Verification items for the finished model (mm, model axes). A direction names the side the tool comes from. Coordinates: 2 decimals unless noted, no trailing zeros. Order: outer loops, then holes, each group sorted by start corner. A loop starts at its lowest first (then second) coordinate and runs counter-clockwise, first axis right, second up.
Q1. Cross-section at C-C, the plane x = 1.1. Count the separate pieces of the cut face and the enclosed holes in it, and give its area (3 significant figures).
Q2. Draft check along Z on faces 1 (the flat face through (2, -65, -40)), 2 (the flat face through (2, -39, 65)), 3 (the cylindrical face through (2, -64, -63)), 4 (the cylindrical face through (1.972, -41.777, 22.704)). Enter one of: pulls with the +Z half, pulls with the -Z half, needs draft (parallel to the pull), parting line crosses it, or undercut.
Q3. Depth check by flat-ended pin: P1, Ø11.5, axis at y = 0, z = -55, coming from the -X side; P2, Ø2, axis at x = 2.5, y = 35, coming from the +Z side; P3, Ø2, axis at x = 1.5, z = -19, coming from the -Y side; P4, Ø1.5, axis at x = 0.5, z = 17, coming from the +Y side. Enter the tip coordinate at first touch or a pass-through.
Q4. Thickness scan on line 1 (Y direction, x = 0.3, z = 36); line 2 (Y direction, x = 0.6, z = 37); line 3 (Y direction, x = 2.45, z = -55). Record the ranges inside material, lowest first.
Q5. Set-up check for faces 5 (the cylindrical face through (1.97, 16.34, 66.02)), 6 (the cylindrical face through (1.972, 3.864, 66.328)), 7 (the cylindrical face through (1.972, 63.963, -17.347)), 8 (the cylindrical face through (1.972, -63.905, -17.274)): record each of +Z, -Z, +X, -X, +Y, -Y from which the full face is reachable in a straight line by a thin tool's end or side.
Q6. Cross-section at D-D, the plane z = 10. Record the boundary of the cut face in (x, y), and give its area (3 significant figures).
Q7. Cross-section at A-A, the plane y = 30. Record the boundary of the cut face in (x, z).
Q8. Cross-section at B-B, the plane y = 53.5. Record the boundary of the cut face in (x, z).
from build123d import *

# Parameters (mm, degrees)
F1_DEPTH = 4


with BuildPart() as f1:
    # F0 (on Right) → F1 (new body)
    with BuildSketch(Plane.YZ):
        with BuildLine():
            Line((-19.364917, 65), (-60, 65))
            ThreePointArc((-60, 65), (-63.535534, 63.535534), (-65, 60))
            Line((-65, 60), (-65, 20.396078))
            ThreePointArc((-65, 20.396078), (-63.933979, 17.310011), (-61.190476, 15.539869))
            ThreePointArc((-61.190476, 15.539869), (-49, 0), (-61.190476, -15.539869))
            ThreePointArc((-61.190476, -15.539869), (-63.933979, -17.310011), (-65, -20.396078))
            Line((-65, -20.396078), (-65, -60))
            ThreePointArc((-65, -60), (-63.535534, -63.535534), (-60, -65))
            Line((-60, -65), (60, -65))
            ThreePointArc((60, -65), (63.535534, -63.535534), (65, -60))
            Line((65, -60), (65, -20.396078))
            ThreePointArc((65, -20.396078), (63.933979, -17.310011), (61.190476, -15.539869))
            ThreePointArc((61.190476, -15.539869), (49, 0), (61.190476, 15.539869))
            ThreePointArc((61.190476, 15.539869), (63.933979, 17.310011), (65, 20.396078))
            Line((65, 20.396078), (65, 60))
            ThreePointArc((65, 60), (63.535534, 63.535534), (60, 65))
            Line((60, 65), (19.364917, 65))
            ThreePointArc((19.364917, 65), (16.303055, 66.047153), (14.523688, 68.75))
            ThreePointArc((14.523688, 68.75), (0, 80), (-14.523688, 68.75))
            ThreePointArc((-14.523688, 68.75), (-16.303055, 66.047153), (-19.364917, 65))
        make_face()
        with BuildLine():
            ThreePointArc((-21.664404, -22.924985), (-22.924985, -41.975206), (-41.975206, -40.714626))
            ThreePointArc((-41.975206, -40.714626), (-45.453544, -16.253883), (-21.664404, -22.924985))
        make_face(mode=Mode.SUBTRACT)
        with BuildLine():
            ThreePointArc((5, -55), (-3.535534, -58.535534), (0, -50))
            ThreePointArc((0, -50), (3.535534, -51.464466), (5, -55))
        make_face(mode=Mode.SUBTRACT)
        with BuildLine():
            ThreePointArc((22.924985, -21.664404), (41.975206, -22.924985), (40.714626, -41.975206))
            ThreePointArc((40.714626, -41.975206), (16.253883, -45.453544), (22.924985, -21.664404))
        make_face(mode=Mode.SUBTRACT)
        with BuildLine():
            ThreePointArc((0, -4.5), (-3.181981, 3.181981), (4.5, 0))
            ThreePointArc((4.5, 0), (3.181981, -3.181981), (0, -4.5))
        make_face(mode=Mode.SUBTRACT)
        with BuildLine():
            ThreePointArc((-22.924985, 21.664404), (-41.975206, 22.924985), (-40.714626, 41.975206))
            ThreePointArc((-40.714626, 41.975206), (-16.253883, 45.453544), (-22.924985, 21.664404))
        make_face(mode=Mode.SUBTRACT)
        with BuildLine():
            ThreePointArc((21.664404, 22.924985), (22.924985, 41.975206), (41.975206, 40.714626))
            ThreePointArc((41.975206, 40.714626), (45.453544, 16.253883), (21.664404, 22.924985))
        make_face(mode=Mode.SUBTRACT)
        with BuildLine():
            ThreePointArc((-5, 71), (0, 76), (5, 71))
            ThreePointArc((5, 71), (4.892932, 69.97082), (4.576315, 68.985716))
            ThreePointArc((4.576315, 68.985716), (3.859883, 66.289083), (4, 63.502423))
            ThreePointArc((4, 63.502423), (4.786744, 58.307337), (4.999482, 53.057325))
            ThreePointArc((4.999482, 53.057325), (0, 48.129323), (-4.999482, 53.057325))
            ThreePointArc((-4.999482, 53.057325), (-4.786744, 58.307337), (-4, 63.502423))
            ThreePointArc((-4, 63.502423), (-3.859883, 66.289083), (-4.576315, 68.985716))
            ThreePointArc((-4.576315, 68.985716), (-4.892932, 69.97082), (-5, 71))
        make_face(mode=Mode.SUBTRACT)
    extrude(amount=F1_DEPTH)


solid = f1.part
Check values:
1. separate pieces: 1
1. enclosed holes: 7
1. area: 12,800 mm2
2. face 1: needs draft
2. face 2: pulls with the +Z half
2. face 3: pulls with the -Z half
2. face 4: undercut
3. P1: stops at x = 0
3. P2: stops at z = 65
3. P3: stops at y = -64.98
3. P4: stops at y = 64.24
4. line 1: y = -65 to -44.66, -12.6 to 18.98, 47.68 to 65
4. line 2: y = -65 to -44.29, -12.65 to 19.35, 46.89 to 65
4. line 3: y = -65 to -5, 5 to 65
5. face 5: +Z, +X, -X, +Y
5. face 6: +X, -X
5. face 7: +X, -X, +Y
5. face 8: +X, -X, -Y
6. outline: (0, -52.51) - (4, -52.51) - (4, 52.51) - (0, 52.51) - close
6. area: 420 mm2
7. outline: (0, -65) - (4, -65) - (4, -50.25) - (0, -50.25) - close; (0, -18.44) - (4, -18.44) - (4, 13.76) - (0, 13.76) - close; (0, 45.2) - (4, 45.2) - (4, 65) - (0, 65) - close
8. outline: (0, -65) - (4, -65) - (4, -11.12) - (0, -11.12) - close; (0, 11.12) - (4, 11.12) - (4, 65) - (0, 65) - close
